The drawing under review shows one solid part. Ordinate dimensions are in mm from its lowest x, y, z. Coordinates: 2 decimals unless noted, no trailing zeros. Order: outer loops, then holes, each group sorted by start corner. A loop starts at its lowest first (then second) coordinate and runs counter-clockwise, first axis right, second up. Notation, with made-up numbers: (24, 72.25) -> (59, 72.25) arc R24 cw to (59, 103.25) -> close; hole circle Ø3 at (76.25, 61). An arc over 180 degrees is marked (long way). Use a Markdown table: item, result. Add a question column.
Q1. Add section D-D (y = 3). State the section outline as (x, z) points.
Q2. Insertion check: pin 1 (7 mm diameter, centred on y = 28.5, z = 66.5, fed in from +X); pin 2 (10 mm diameter, centred on x = 103.5, z = 85, fed in from -Y); pin 3 (12 mm diameter, centred on x = 196, y = 22, fed in from +Z). Each pin has a flat end and moves straight along its axis. Give the tip position at first contact, or say it passes through.
Q3. Add section C-C (z = 61). State the section outline as (x, y) points, then the cut area to 3 significant figures.
Q4. Add section A-A (x = 257). State the section outline as (y, z) points.
Q5. Add section B-B (x = 224.5). State the section outline as (y, z) points, then the cut area to 3 significant figures.
Q6. Wall thickness on probe 1 along Y at (x, z) = (128, 168); probe 2 along Z at (x, y) = (40, 27); probe 3 along Z at (x, y) = (249, 26): over which ranges is each line inside the solid? List them lowest first.
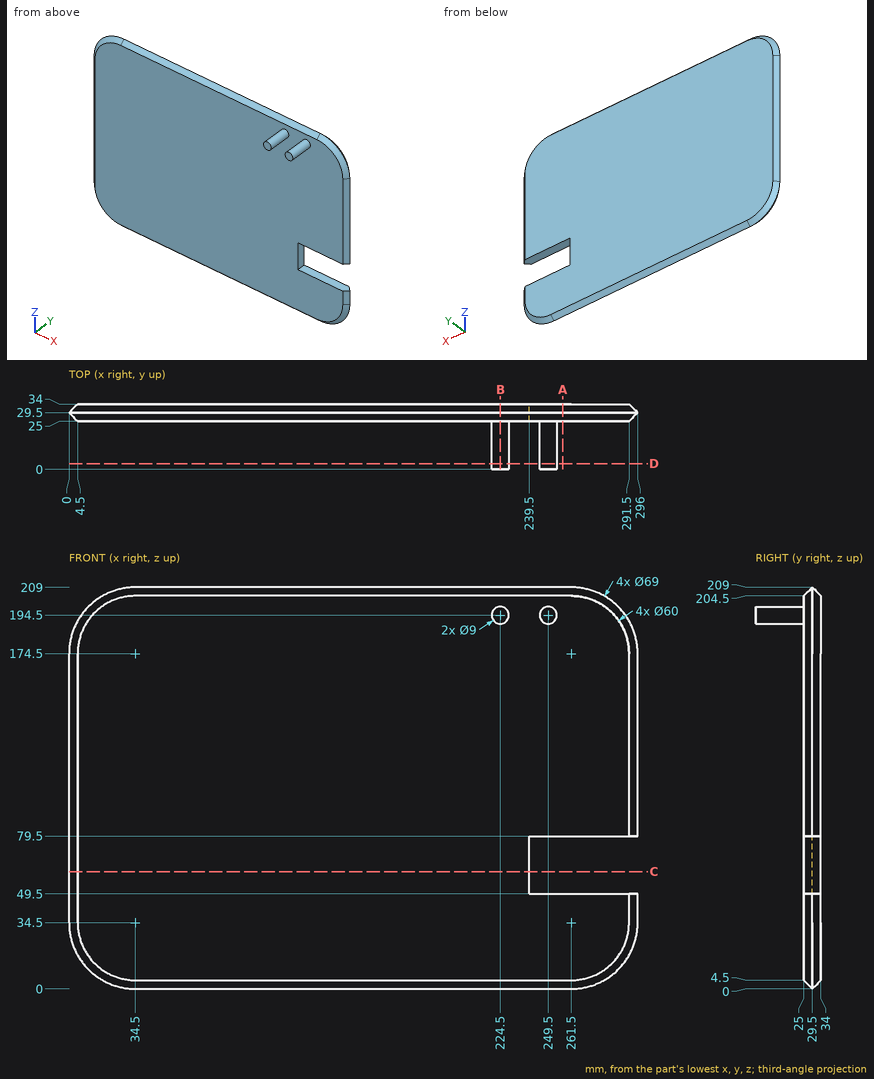
Established:
| question | item | result |
|---|---|---|
| 1 | outline | circle Ø9 at (224.5, 194.5); circle Ø9 at (249.5, 194.5) |
| 2 | pin 1 | x = 239.5 |
| 2 | pin 2 | y = 25 |
| 2 | pin 3 | z = 207.5 |
| 3 | outline | (0, 29.5) -> (4.5, 25) -> (239.5, 25) -> (239.5, 34) -> (4.5, 34) -> close |
| 3 | area | 2,140 mm^2 |
| 4 | outline | (25, 4.5) -> (29.5, 0) -> (34, 4.5) -> (34, 49.5) -> (25, 49.5) -> close; (25, 79.5) -> (34, 79.5) -> (34, 204.5) -> (29.5, 209) -> (25, 204.5) -> close |
| 5 | outline | (0, 190) -> (25, 190) -> (25, 4.5) -> (29.5, 0) -> (34, 4.5) -> (34, 204.5) -> (29.5, 209) -> (25, 204.5) -> (25, 199) -> (0, 199) -> close |
| 5 | area | 2,070 mm^2 |
| 6 | probe 1 | 25 to 34 |
| 6 | probe 2 | 2.5 to 206.5 |
| 6 | probe 3 | 3.5 to 49.5, 79.5 to 205.5 |
